Can you work these out from the drawing? Everything is in mm from the part's minimum corner. A direction names the side the tool comes from. Coordinates: 2 decimals unless noted, no trailing zeros. Order: outer loops, then holes, each group sorted by start corner. A loop starts at its lowest first (then second) coordinate and runs counter-clockwise, first axis right, second up. Notation, with made-up numbers: (43, 21) -> (51, 21) arc R32 ccw to (51, 48) -> close; hole circle Ø11 at (34, 65). An arc over 180 degrees is marked (long way). Use a Markdown table: item, result. Add a question column.
1) Thinking about a two-plate mould opening in Z: for the marked faces 1, 2, 3 and 4, which applies, +Z half, -Z half, draft (parallel to the pull), parting line (faces both ways), or undercut?
2) Will these pins go through, and if not, where does the flat tip stop? pin 1 Ø8 at (y, z) = (29, 15) entering from +X; pin 2 Ø6 at (x, z) = (37.5, 14.5) entering from -Y (1 decimal); pin 3 Ø22.5 at (x, z) = (20, 41) entering from +Y.
3) Which directions (+Z, -Z, +X, -X, +Y, -Y) give clear straight access to the entire face, cutting with the end or side of a thin tool? Please do the marked faces 5, 6, 7 and 8.
4) If we section it at D-D (z = 6): Write out the boundary of the cut face in (x, y), plus the area to 3 significant figures.
5) If we section it at A-A (y = 33): Write out the boundary of the cut face in (x, z) (1 decimal).
6) If I drill on L1, parallel to Z at x = 44, y = 30.5; L2, parallel to X at y = 28, z = 20.5; L3, parallel to X at y = 17, z = 26.5, over which ranges is the centre line in solid material (lowest first)? Write a range as [from, to].
7) If we section it at B-B (z = 48): Write out the boundary of the cut face in (x, y), plus the area to 3 significant figures.
8) If we section it at C-C (x = 15): Write out the boundary of the cut face in (y, z).
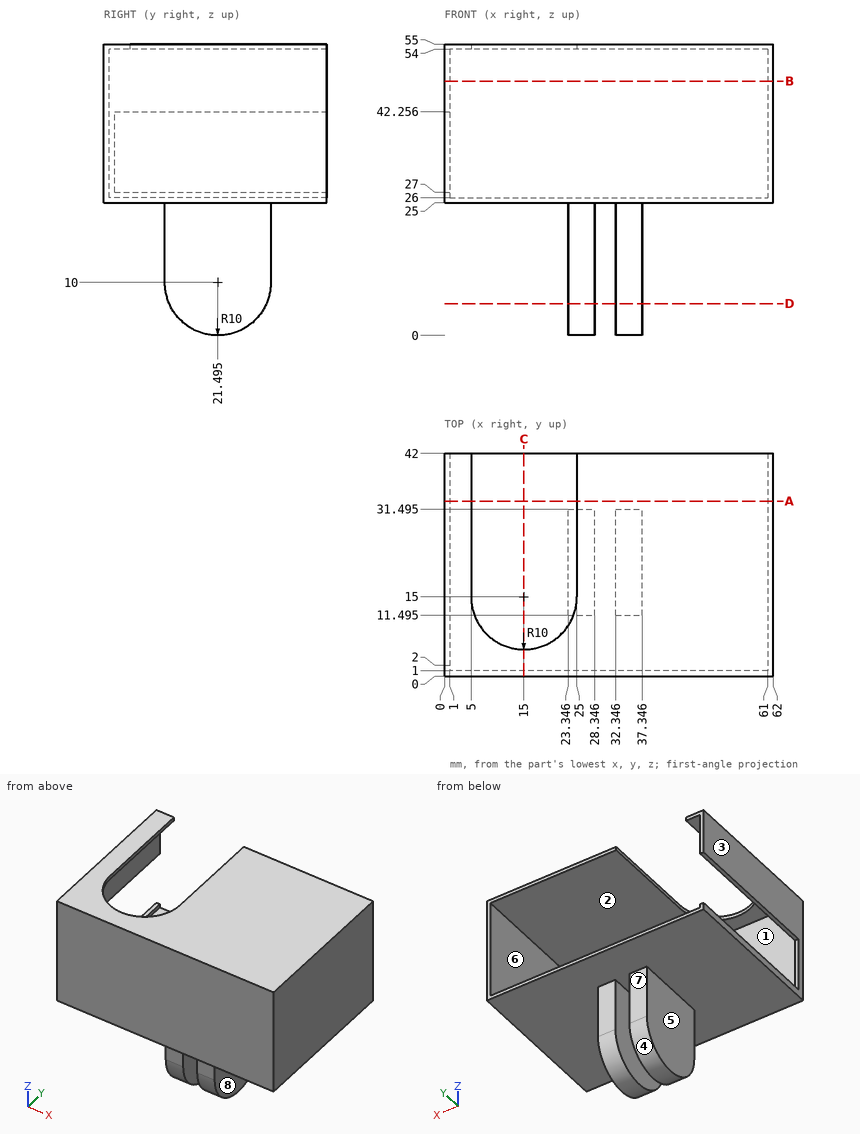
Answer sheet:
| question | item | result |
|---|---|---|
| 1 | face 1 | undercut |
| 1 | face 2 | undercut |
| 1 | face 3 | draft |
| 1 | face 4 | -Z half |
| 2 | pin 1 | x = 37.35 |
| 2 | pin 2 | y = 11.5 |
| 2 | pin 3 | y = 1 |
| 3 | face 5 | -Z, -X, +Y, -Y |
| 3 | face 6 | +Y |
| 3 | face 7 | -Z, +X, -X, +Y |
| 3 | face 8 | -Z, +X, +Y, -Y |
| 4 | outline | (23.35, 12.33) -> (28.35, 12.33) -> (28.35, 30.66) -> (23.35, 30.66) -> close; (32.35, 12.33) -> (37.35, 12.33) -> (37.35, 30.66) -> (32.35, 30.66) -> close |
| 4 | area | 183 mm2 |
| 5 | outline | (0, 25) -> (62, 25) -> (62, 55) -> (25, 55) -> (25, 54) -> (61, 54) -> (61, 26) -> (1, 26) -> (1, 27) -> (0, 27) -> close; (0, 42.3) -> (1, 42.3) -> (1, 54) -> (5, 54) -> (5, 55) -> (0, 55) -> close |
| 6 | L1 | [25, 26], [54, 55] |
| 6 | L2 | [23.35, 28.35], [32.35, 37.35] |
| 6 | L3 | [0, 1], [61, 62] |
| 7 | outline | (0, 0) -> (62, 0) -> (62, 42) -> (61, 42) -> (61, 1) -> (1, 1) -> (1, 42) -> (0, 42) -> close |
| 7 | area | 144 mm2 |
| 8 | outline | (0, 25) -> (42, 25) -> (42, 26) -> (1, 26) -> (1, 54) -> (5, 54) -> (5, 55) -> (0, 55) -> close |
